Could you check a few things on this model? Use its own coordinates, in mm. A direction names the side the tool comes from. Give positions to 0.01 mm unless a question says otherwise; leave off trailing zeros. Loops run counter-clockwise (first coordinate to the right, second up) from the corner with the lowest first, then second, coordinate; pieces in that order, holes last. Notation, with made-up numbers: (41.25, -26) - (82.25, -26) arc R23 ccw to (82.25, -6) - close; hole circle Ø2 at (45, -10). An arc over 180 degrees is marked (long way). One line per item, written item: value. Start each with the question number.
Q1. For faces 5 (the face through (-10.61, 1.97, 50.73)), 6 (the face through (8, 2, -44.25)), 7 (the face through (-9.573, 1.972, -41.17)), which set-ups out of +Z, -Z, +X, -X, +Y, -Y let a thin tool reach every point of the face, with its end or its side?
Q2. If I drill on line 1 (Z direction, x = -4.25, y = 2); line 2 (X direction, y = 2.3, z = 49.25); line 3 (Z direction, x = 9, y = 1.8), over which ranges is the centre line in solid material (lowest first)? Write a range as from..to.
Q3. I'm going to push a flat-ended pin straight in: P1, Ø2, axis at y = 3, z = -7.5, coming from the +X side. Where does the tip first touch, or does it pass through?
Q4. If we mould it in two halves opening along X, with no side actions, what happens to faces 1 (the face through (-5.164, 1.972, 16.445)), 2 (the face through (9, 2, -48)), 3 (the face through (8, 2, 44.25)), 4 (the face through (2.24, 1.97, -42.75))? For each: released by +X, released by -X, zero draft, split by the parting line, or undercut.
Q5. I want a section at B-B (y = 0.95). Please give me the cut outline in (x, z) (3 decimals).
Q6. I want a section at C-C (z = -12.5). Please give me the cut outline in (x, y).
Q7. I want a section at A-A (z = 49.25). Please give me the cut outline in (x, y).
```python
from build123d import *

# Parameters (mm, degrees)
SKETCH1_R           = 1.6
BOSS_EXTRUDE1_DEPTH = 4


with BuildPart() as part:
    # Sketch1 → Boss-Extrude1 (new body)
    with BuildSketch(Plane(origin=(0, 0, 0), x_dir=(1, 0, 0), z_dir=(0, 1, 0))):
        with BuildLine():
            Line((10, 54.25), (-10, 54.25))
            ThreePointArc((-10, 54.25), (-14.611555285, 51.182241665), (-13.564255704, 45.74342314))
            Line((-13.564255704, 45.74342314), (-10.625744296, 42.75657686))
            ThreePointArc((-10.625744296, 42.75657686), (-9.562836802, 41.14456083), (-9.19, 39.25))
            Line((-9.19, 39.25), (-9.19, -39.25))
            ThreePointArc((-9.19, -39.25), (-9.562836802, -41.14456083), (-10.625744296, -42.75657686))
            Line((-10.625744296, -42.75657686), (-13.564255704, -45.74342314))
            ThreePointArc((-13.564255704, -45.74342314), (-14.611555285, -51.182241665), (-10, -54.25))
            Line((-10, -54.25), (10, -54.25))
            ThreePointArc((10, -54.25), (15, -49.25), (10, -44.25))
            Line((10, -44.25), (5.81, -44.25))
            ThreePointArc((5.81, -44.25), (2.274466094, -42.785533906), (0.81, -39.25))
            Line((0.81, -39.25), (0.81, 39.25))
            ThreePointArc((0.81, 39.25), (2.274466094, 42.785533906), (5.81, 44.25))
            Line((5.81, 44.25), (10, 44.25))
            ThreePointArc((10, 44.25), (15, 49.25), (10, 54.25))
        make_face()
        with Locations(Location((-10, 49.25, 0), (0, 0, 270))):
            Circle(SKETCH1_R, mode=Mode.SUBTRACT)
        with Locations(Location((10, 49.25, 0), (0, 0, 270))):
            Circle(SKETCH1_R, mode=Mode.SUBTRACT)
        with Locations(Location((-4.19, -17.715, 0), (0, 0, 270))):
            Circle(SKETCH1_R, mode=Mode.SUBTRACT)
        with Locations(Location((-4.19, 17.715, 0), (0, 0, 270))):
            Circle(SKETCH1_R, mode=Mode.SUBTRACT)
        with Locations(Location((10, -49.25, 0), (0, 0, 270))):
            Circle(SKETCH1_R, mode=Mode.SUBTRACT)
        with Locations(Location((-10, -49.25, 0), (0, 0, 270))):
            Circle(SKETCH1_R, mode=Mode.SUBTRACT)
    extrude(amount=BOSS_EXTRUDE1_DEPTH)


solid = part.part
```
Worked answers:
1. face 5: +Y, -Y
1. face 6: +X, +Y, -Y
1. face 7: -X, +Y, -Y
2. line 1: z = -54.25..-19.31, -16.12..16.12, 19.31..54.25
2. line 2: x = -15..-11.6, -8.4..8.4, 11.6..15
2. line 3: z = -54.25..-50.5, -48..-44.25, 44.25..48, 50.5..54.25
3. P1: stops at x = 0.81
4. face 1: undercut
4. face 2: undercut
4. face 3: zero draft
4. face 4: released by +X
5. outline: (-13.564, -45.743) arc R5 ccw to (-10, -54.25) - (10, -54.25) arc R5 ccw to (10, -44.25) - (5.81, -44.25) arc R5 cw to (0.81, -39.25) - (0.81, 39.25) arc R5 cw to (5.81, 44.25) - (10, 44.25) arc R5 ccw to (10, 54.25) - (-10, 54.25) arc R5 ccw to (-13.564, 45.743) - (-10.626, 42.757) arc R5 cw to (-9.19, 39.25) - (-9.19, -39.25) arc R5 cw to (-10.626, -42.757) - close; hole circle Ø3.2 at (-10, -49.25); hole circle Ø3.2 at (-10, 49.25); hole circle Ø3.2 at (-4.19, -17.715); hole circle Ø3.2 at (-4.19, 17.715); hole circle Ø3.2 at (10, -49.25); hole circle Ø3.2 at (10, 49.25)
6. outline: (-9.19, 0) - (0.81, 0) - (0.81, 4) - (-9.19, 4) - close
7. outline: (-15, 0) - (-11.6, 0) - (-11.6, 4) - (-15, 4) - close; (-8.4, 0) - (8.4, 0) - (8.4, 4) - (-8.4, 4) - close; (11.6, 0) - (15, 0) - (15, 4) - (11.6, 4) - close
